Check sheet for the modelled part. Datum: model origin and axes. Units: mm. Give positions to 0.01 mm unless a question says otherwise; leave off trailing zeros. Loops run counter-clockwise (first coordinate to the right, second up) from the corner with the lowest first, then second, coordinate; pieces in that order, holes last. Notation, with made-up numbers: (66, 34.5) - (125, 34.5) arc R4 ccw to (125, 39.5) - close; hole circle Ø2 at (-29, 18). An arc over 180 degrees is marked (long way). Use one line per item in the form item = value.
from build123d import *

# Parameters (mm, degrees)
EXTRUDE_1_DEPTH     = 5
FILLET_1_R          = 1
SKETCH_2_R          = 2
CUT_EXTRUDE_1_DEPTH = 10
FILLET_2_R          = 1


with BuildPart() as part:
    # Эскиз1 → Бобышка-Вытянуть1 (new body)
    with BuildSketch(Plane(origin=(0, 0, 0), x_dir=(1, 0, 0), z_dir=(0, 1, 0))):
        Polygon((13.5, 0), (6.75, 11.691342951), (-6.75, 11.691342951), (-13.5, 0), (-6.75, -11.691342951), (6.75, -11.691342951), align=None)
    extrude(amount=EXTRUDE_1_DEPTH)

    # Скругление1
    fillet_1_edges = [part.edges().sort_by_distance(p)[0] for p in [
        (6.75, 2.5, 11.691342951),
        (-6.75, 2.5, 11.691342951),
        (-13.5, 2.5, 0),
        (-6.75, 2.5, -11.691342951),
        (6.75, 2.5, -11.691342951),
        (13.5, 2.5, 0),
    ]]
    fillet(fillet_1_edges, radius=FILLET_1_R)

    # Эскиз2 → Вырез-Вытянуть1 (cut)
    with BuildSketch(Plane(origin=(0, 5, 0), x_dir=(1, 0, 0), z_dir=(0, 1, 0))):
        with Locations(Location((5, 8.660254038, 0), (0, 0, 270))):
            Circle(SKETCH_2_R)
        with Locations((8.660254038, -5)):
            Circle(SKETCH_2_R)
        with Locations(Location((-5, -8.660254038, 0), (0, 0, 270))):
            Circle(SKETCH_2_R)
        with Locations((-8.660254038, 5)):
            Circle(SKETCH_2_R)
    extrude(amount=-CUT_EXTRUDE_1_DEPTH, mode=Mode.SUBTRACT)

    # Скругление2
    fillet_2_edges = [part.edges().sort_by_distance(p)[0] for p in [
        (-9.591296191, 2.5, -6.770073588),
        (-10.658703809, 2.5, -4.921269363),
        (9.591296191, 2.5, 6.770073588),
        (10.658703809, 2.5, 4.921269363),
    ]]
    fillet(fillet_2_edges, radius=FILLET_2_R)


solid = part.part
Item 1: Section check C-C on z = 7.25. Record the boundary of the cut face in (x, y).
Answer block:
outline = (-9.31, 0) - (-6.42, 0) - (-6.42, 5) - (-9.31, 5) - close; (-3.58, 0) - (8.58, 0) - (8.58, 5) - (-3.58, 5) - close
Item 2: Mould release check, pull along Z, two halves, no side actions. Record for faces 1 (the face through (-6.95, 2.54, -3.96)), 2 (the face through (-13.345, 2.535, -0.007)), 3 (the face through (6.67, 2.54, 11.56)): released by +Z, released by -Z, zero draft, split by the parting line, or undercut.
Answer block:
face_1 = undercut
face_2 = split by the parting line
face_3 = released by +Z
Item 3: Thickness scan on L1, parallel to X at y = 1.35, z = -7; L2, parallel to Z at x = 6, y = 1.45; L3, parallel to X at y = 2.4, z = -3.25. Record the ranges inside material, lowest first.
Answer block:
L1 = -8.29 to 3.88, 6.12 to 9.46
L2 = -11.69 to -10.39, -6.93 to 11.69
L3 = -11.62 to -9.63, -7.69 to 11.62
Item 4: Gauge pin test, flat ends, axial feed: P1, Ø5, axis at x = -3, z = 7, coming from the -Y side; P2, Ø2, axis at y = 2, z = -5.5, coming from the +X side; P3, Ø2, axis at y = 2, z = -1.5, coming from the -X side; P4, Ø1.5, axis at y = 2, z = 4, coming from the -X side. Record the tip position at first contact, or that the pin passes through.
Answer block:
P1 = 0
P2 = 10.9
P3 = -13.21
P4 = -11.62
Item 5: Section check A-A on x = -5. Record the boundary of the cut face in (y, z).
Answer block:
outline = (0, -11.69) - (5, -11.69) - (5, 6.66) - (0, 6.66) - close; (0, 10.66) - (5, 10.66) - (5, 11.69) - (0, 11.69) - close
Item 6: Section check B-B on y = 2.75. Record the boundary of the cut face in (x, z), then the cut area to 3 significant figures.
Answer block:
outline = (-13.21, -0.5) - (-11.58, -3.32) arc R1 ccw to (-10.03, -3.55) arc R2 cw (long way) to (-8.09, -6.92) arc R1 ccw to (-8.67, -8.37) - (-7.04, -11.19) arc R1 ccw to (-6.17, -11.69) - (6.17, -11.69) arc R1 ccw to (7.04, -11.19) - (13.21, -0.5) arc R1 ccw to (13.21, 0.5) - (11.58, 3.32) arc R1 ccw to (10.03, 3.55) arc R2 cw (long way) to (8.09, 6.92) arc R1 ccw to (8.67, 8.37) - (7.04, 11.19) arc R1 ccw to (6.17, 11.69) - (-6.17, 11.69) arc R1 ccw to (-7.04, 11.19) - (-13.21, 0.5) arc R1 ccw to start; hole circle Ø4 at (-5, 8.66); hole circle Ø4 at (5, -8.66)
area = 422 mm2
Item 7: Section check D-D on z = 2. Record the boundary of the cut face in (x, y).
Answer block:
outline = (-12.35, 0) - (12.35, 0) - (12.35, 5) - (-12.35, 5) - close
